Read the model definition and answer for the solid it produces. Units are mm, in the model's axes. A direction names the side the tool comes from. Coordinates: 2 decimals unless noted, no trailing zeros. Loops run counter-clockwise (first coordinate to the right, second up) from the corner with the lowest first, then second, coordinate; pieces in that order, holes last. Notation, with made-up numbers: (81.25, 23) -> (124.25, 23) arc R36 ccw to (124.25, 61) -> close; hole circle Ø9 at (68.25, 16). An arc over 180 degrees is marked (long way). Answer in a Markdown table with one row per item.
```python
from build123d import *

# Parameters (mm, degrees)
EXTRUDE_1_DEPTH                 = 60.5
SHELL_1_T                       = -2.5
EXTRUDE_3_DEPTH                 = 4.55
CUT_EXTRUDE_1_REACH             = 237.14
SKETCH_7_W                      = 1.95
SKETCH_7_H                      = 39
CUT_EXTRUDE_1_DIRECTION_2_REACH = 237.14
SKETCH_8_W                      = 59
SKETCH_8_H                      = 58
SKETCH_8_R                      = 21
EXTRUDE_5_DEPTH                 = 3
HOLE_START                      = 77.45
HOLE_WIZARD_M3_1_OUTLINE_R      = 1.25
HOLE_WIZARD_M3_1_DEPTH          = 7.55
PATTERN_LINEAR_1_COUNT          = 2
PATTERN_LINEAR_1_PITCH          = 45
PATTERN_LINEAR_1_COUNT_DIR2     = 2
PATTERN_LINEAR_1_PITCH_DIR2     = 44
SKETCH_13_W                     = 64
SKETCH_13_H                     = 60.5
SKETCH_13_R                     = 21
EXTRUDE_6_DEPTH                 = 3
HOLE_WIZARD_M3_2_REACH          = 146.84
HOLE_WIZARD_M3_2_BORE_R         = 1.25
PATTERN_LINEAR_2_COUNT          = 2
PATTERN_LINEAR_2_PITCH          = 45
PATTERN_LINEAR_2_COUNT_DIR2     = 2
PATTERN_LINEAR_2_PITCH_DIR2     = 44
CUT_EXTRUDE_2_REACH             = 240.449
SKETCH_16_R                     = 15
HOLE_WIZARD_M3_3_REACH          = 240.449
HOLE_WIZARD_M3_3_BORE_R         = 1.25
PATTERN_LINEAR_3_COUNT          = 2
PATTERN_LINEAR_3_PITCH          = 40
PATTERN_LINEAR_3_COUNT_DIR2     = 2
PATTERN_LINEAR_3_PITCH_DIR2     = 36.5
EXTRUDE_7_DEPTH                 = 58
CUT_EXTRUDE_4_DEPTH             = 12
CUT_EXTRUDE_5_REACH             = 237.925
SKETCH_22_W                     = 6.65
SKETCH_22_H                     = 14
EXTRUDE_8_DEPTH                 = 2


# Read off the part's stored shape, not the designer's step: M3 螺纹孔1
with BuildPart() as part:
    # 草图2 → 凸台-拉伸1 (new body)
    with BuildSketch(Plane(origin=(0, 0, 0), x_dir=(1, 0, 0), z_dir=(0, 1, 0))):
        Polygon((0, -32), (82.5, -32), (85, -41.313840204), (161.143914202, -96.432841737), (209.519633633, -29.6044064), (194.938884105, -19.049703979), (184.090995505, -34.035474327), (122.527830831, 10.528824785), (85, 32), (0, 32), align=None)
    extrude(amount=EXTRUDE_1_DEPTH)

    # 抽壳1
    shell_1_openings = [part.faces().sort_by_distance(p)[0] for p in [
        (97.534213711, 60.5, 20.40382731),
    ]]
    offset(amount=SHELL_1_T, openings=shell_1_openings, kind=Kind.INTERSECTION)

    # 草图5 → 凸台-拉伸3 (add)
    with BuildSketch(Plane.ZY.offset(-85)):
        Polygon((-32, 60.5), (-32, 2.5), (32, 2.5), (32, 60.5), (8.5, 60.5), (8.5, 21.5), (-8.5, 21.5), (-8.5, 60.5), align=None)
    extrude(amount=EXTRUDE_3_DEPTH)

    # 切除-拉伸1: up to this face of the body (flat: up to its plane)
    cut_extrude_1_end = Plane(part.part.faces().sort_by_distance((41.475, 31.5, 29.5))[0])
    # 草图7 → 切除-拉伸1 (cut, up to the picked face)
    with BuildSketch(Plane(origin=(0, 0, 8.5), x_dir=(-1, 0, 0), z_dir=(0, 0, -1)), mode=Mode.PRIVATE) as cut_extrude_1_sk1:
        with Locations((-82.725, 41)):
            Rectangle(SKETCH_7_W, SKETCH_7_H)
    cut_extrude_1_tool1 = split(extrude(cut_extrude_1_sk1.sketch, amount=-CUT_EXTRUDE_1_REACH, mode=Mode.PRIVATE), bisect_by=cut_extrude_1_end, keep=Keep.BOTH, mode=Mode.PRIVATE)
    add(cut_extrude_1_tool1.solids().sort_by(Axis((82.725, 41, 8.5), (0, 0, 1)))[0], mode=Mode.SUBTRACT)

    # 切除-拉伸1 direction 2: up to this face of the body (flat: up to its plane)
    cut_extrude_1_direction_2_end = Plane(part.part.faces().sort_by_distance((41.475, 31.5, -29.5))[0])
    # 草图7 → 切除-拉伸1 direction 2 (cut, up to the picked face)
    with BuildSketch(Plane(origin=(0, 0, 8.5), x_dir=(-1, 0, 0), z_dir=(0, 0, -1)), mode=Mode.PRIVATE) as cut_extrude_1_direction_2_sk1:
        with Locations((-82.725, 41)):
            Rectangle(SKETCH_7_W, SKETCH_7_H)
    cut_extrude_1_direction_2_tool1 = split(extrude(cut_extrude_1_direction_2_sk1.sketch, amount=CUT_EXTRUDE_1_DIRECTION_2_REACH, mode=Mode.PRIVATE), bisect_by=cut_extrude_1_direction_2_end, keep=Keep.BOTH, mode=Mode.PRIVATE)
    add(cut_extrude_1_direction_2_tool1.solids().sort_by(Axis((82.725, 41, 8.5), (0, 0, -1)))[0], mode=Mode.SUBTRACT)

    # 草图8 → 凸台-拉伸5 (add)
    with BuildSketch(Plane.ZY.offset(-80.45)):
        with Locations((0, 31.5)):
            Rectangle(SKETCH_8_W, SKETCH_8_H)
        with Locations(Location((0, 31.5, 0), (0, 0, 113.876207731))):
            Circle(SKETCH_8_R, mode=Mode.SUBTRACT)
    extrude(amount=EXTRUDE_5_DEPTH)

    # M3 螺纹孔1 outline → M3 螺纹孔1 (cut)
    with BuildSketch(Plane.YZ.offset(HOLE_START)):
        with Locations((53.5, -22.5)):
            Circle(HOLE_WIZARD_M3_1_OUTLINE_R)
    hole_wizard_m3_1 = extrude(amount=HOLE_WIZARD_M3_1_DEPTH, mode=Mode.SUBTRACT)

    # 阵列(线性)1: Hole Wizard M3 _1 2 × 2
    with Locations(*[(0, -j * PATTERN_LINEAR_1_PITCH_DIR2, i * PATTERN_LINEAR_1_PITCH) for i in range(PATTERN_LINEAR_1_COUNT) for j in range(PATTERN_LINEAR_1_COUNT_DIR2) if (i, j) != (0, 0)]):
        add(hole_wizard_m3_1, mode=Mode.SUBTRACT)

    # 草图13 → 凸台-拉伸6 (add)
    with BuildSketch(Plane(origin=(75.397730804, 0, 54.578854835), x_dir=(0.5863723567357906, 0, -0.8100416404457952), z_dir=(0.8100416404457952, 0, 0.5863723567357906))):
        with Locations((48.375719431, 30.25)):
            Rectangle(SKETCH_13_W, SKETCH_13_H)
        with Locations((48.375719431, 30.25)):
            Circle(SKETCH_13_R, mode=Mode.SUBTRACT)
    extrude(amount=EXTRUDE_6_DEPTH)

    # M3 螺纹孔2 bore (on position points) → M3 螺纹孔2 (cut, up to next)
    with BuildSketch(Plane(origin=(93.00066231, 53.5, 35.37756169), x_dir=(-0.586372356736, 0, 0.810041640446), z_dir=(0.810041640446, 0, 0.586372356736)), mode=Mode.PRIVATE) as hole_wizard_m3_2_sk1:
        Circle(HOLE_WIZARD_M3_2_BORE_R)
    hole_wizard_m3_2_tool1 = extrude(hole_wizard_m3_2_sk1.sketch, amount=-HOLE_WIZARD_M3_2_REACH, mode=Mode.PRIVATE) & part.part
    hole_wizard_m3_2 = hole_wizard_m3_2_tool1.solids().sort_by_distance((93.000662, 53.5, 35.377562))[0]
    add(hole_wizard_m3_2, mode=Mode.SUBTRACT)

    # 阵列(线性)2: Hole Wizard M3 _2 2 × 2
    with Locations(*[Vector(0.5863723567357906, 0, -0.8100416404457951) * (i * PATTERN_LINEAR_2_PITCH) + Vector(0, -1, 0) * (j * PATTERN_LINEAR_2_PITCH_DIR2) for i in range(PATTERN_LINEAR_2_COUNT) for j in range(PATTERN_LINEAR_2_COUNT_DIR2) if (i, j) != (0, 0)]):
        add(hole_wizard_m3_2, mode=Mode.SUBTRACT)

    # 草图16 → 切除-拉伸2 (cut, up to next)
    with BuildSketch(Plane.ZY, mode=Mode.PRIVATE) as cut_extrude_2_sk1:
        with Locations((0, 30.25)):
            Circle(SKETCH_16_R)
    cut_extrude_2_tool1 = extrude(cut_extrude_2_sk1.sketch, amount=-CUT_EXTRUDE_2_REACH, mode=Mode.PRIVATE) & part.part
    add(cut_extrude_2_tool1.solids().sort_by_distance((0, 30.25, 0))[0], mode=Mode.SUBTRACT)

    # M3 螺纹孔3 bore → M3 螺纹孔3 (cut, up to next)
    with BuildSketch(Plane.ZY, mode=Mode.PRIVATE) as hole_wizard_m3_3_sk1:
        with Locations((-20, 48.5)):
            Circle(HOLE_WIZARD_M3_3_BORE_R)
    hole_wizard_m3_3_tool1 = extrude(hole_wizard_m3_3_sk1.sketch, amount=-HOLE_WIZARD_M3_3_REACH, mode=Mode.PRIVATE) & part.part
    hole_wizard_m3_3 = hole_wizard_m3_3_tool1.solids().sort_by_distance((0, 48.5, -20))[0]
    add(hole_wizard_m3_3, mode=Mode.SUBTRACT)

    # 阵列(线性)3: Hole Wizard M3 _3 2 × 2
    with Locations(*[(0, -j * PATTERN_LINEAR_3_PITCH_DIR2, i * PATTERN_LINEAR_3_PITCH) for i in range(PATTERN_LINEAR_3_COUNT) for j in range(PATTERN_LINEAR_3_COUNT_DIR2) if (i, j) != (0, 0)]):
        add(hole_wizard_m3_3, mode=Mode.SUBTRACT)

    # 草图19 → 凸台-拉伸7 (add)
    with BuildSketch(Plane(origin=(0, 2.5, 0), x_dir=(1, 0, 0), z_dir=(0, 1, 0))):
        Polygon((153.493245308, -82.870402226), (151.147755881, -86.110568788), (160.584740993, -92.941806744), (162.93023042, -89.701640182), (158.880022217, -86.769778399), (158.000463682, -87.984840859), (156.663894976, -87.017326471), (157.543453511, -85.80226401), align=None)
        Polygon((206.02859864, -30.16357961), (201.978390437, -27.231717826), (200.219273367, -29.661842747), (204.269481569, -32.593704531), align=None)
        Polygon((195.498057314, -22.540738972), (200.641821731, -26.264203437), (198.88270466, -28.694328359), (193.738940244, -24.970863893), align=None)
    extrude(amount=EXTRUDE_7_DEPTH)

    # 草图21 → 切除-拉伸4 (cut)
    with BuildSketch(Plane(origin=(0, 60.5, 0), x_dir=(1, 0, 0), z_dir=(0, 1, 0))):
        Polygon((200.219273367, -29.661842747), (201.978390437, -27.231717826), (203.314959144, -28.199232214), (201.555842074, -30.629357136), align=None)
    extrude(amount=-CUT_EXTRUDE_4_DEPTH, mode=Mode.SUBTRACT)

    # 草图22 → 切除-拉伸5 (cut, up to next)
    with BuildSketch(Plane(origin=(9.602269196, 0, -13.265014631), x_dir=(0.810041640445795, 0, 0.5863723567357908), z_dir=(-0.5863723567357908, 0, 0.810041640445795)), mode=Mode.PRIVATE) as cut_extrude_5_sk1:
        with Locations((181.253833284, 12.5)):
            Rectangle(SKETCH_22_W, SKETCH_22_H)
    cut_extrude_5_tool1 = extrude(cut_extrude_5_sk1.sketch, amount=-CUT_EXTRUDE_5_REACH, mode=Mode.PRIVATE) & part.part
    add(cut_extrude_5_tool1.solids().sort_by_distance((156.425422, 12.5, 93.017223))[0], mode=Mode.SUBTRACT)

    # 草图23 → 凸台-拉伸8 (add)
    with BuildSketch(Plane(origin=(0, 60.5, 0), x_dir=(1, 0, 0), z_dir=(0, 1, 0))):
        Polygon((1.25, 30.75), (1.25, -30.75), (83.458724754, -30.75), (86.092274477, -40.561384515), (160.864327597, -94.687324241), (207.774116136, -29.883993005), (195.218470709, -20.795221475), (184.37058211, -35.780991824), (121.849033271, 9.477061724), (84.667685679, 30.75), align=None)
        Polygon((2.5, 29.5), (2.5, -29.5), (84.417449509, -29.5), (87.184548954, -39.808928826), (160.584740993, -92.941806744), (206.02859864, -30.16357961), (195.498057314, -22.540738972), (184.650168714, -37.52650932), (121.170235712, 8.425298663), (84.335371357, 29.5), align=None, mode=Mode.SUBTRACT)
    extrude(amount=EXTRUDE_8_DEPTH)


solid = part.part
```
1. A cutting plane is placed at C-C on x = 137.5. Give the vertices of the cut face in (y, z).
A:
| item | result |
|---|---|
| outline | (0, 0.31) -> (60.5, 0.31) -> (60.5, 1.85) -> (62.5, 1.85) -> (62.5, 3.4) -> (2.5, 3.4) -> (2.5, 76.23) -> (62.5, 76.23) -> (62.5, 77.77) -> (60.5, 77.77) -> (60.5, 79.32) -> (0, 79.32) -> close |
2. A cutting plane is placed at A-A on x = 172.5. Give the vertices of the cut face in (y, z) (3 decimals), and give its area (3 significant figures).
A:
| item | result |
|---|---|
| outline | (0, 25.645) -> (60.5, 25.645) -> (60.5, 27.188) -> (62.5, 27.188) -> (62.5, 28.731) -> (2.5, 28.731) -> (2.5, 76.482) -> (62.5, 76.482) -> (62.5, 78.613) -> (60.5, 78.613) -> (60.5, 80.745) -> (0, 80.745) -> close |
| area | 571 mm2 |
3. Given pin 1 Ø3.5 at (x, z) = (83, 12) entering from +Y; pin 2 Ø2 at (y, z) = (53.5, -22.5) entering from +X; pin 3 Ø8 at (x, y) = (84.5, 36.5) entering from +Z, each flat-ended and moving along its own axis, determine where each tip first touches the part or whether it passes through.
A:
| item | result |
|---|---|
| pin 1 | stops at y = 60.5 |
| pin 2 | stops at x = 103.35 |
| pin 3 | stops at z = 43.85 |
4. A cutting plane is placed at B-B on z = 57.5. Give the vertices of the cut face in (x, y).
A:
| item | result |
|---|---|
| outline | (107.36, 0) -> (189.33, 0) -> (189.33, 60.5) -> (187.78, 60.5) -> (187.78, 62.5) -> (186.24, 62.5) -> (186.24, 2.5) -> (111.62, 2.5) -> (111.62, 62.5) -> (109.49, 62.5) -> (109.49, 60.5) -> (107.36, 60.5) -> close |
5. Find the intervals of material crossed by probe 1 along Z at (x, y) = (80.4, 53.5); probe 2 along X at (y, z) = (15.5, 84); probe 3 along Z at (x, y) = (1, 30), in increasing order.
A:
| item | result |
|---|---|
| probe 1 | z = -32 to -23.75, -21.25 to 21.25, 23.75 to 32 |
| probe 2 | x = 143.97 to 148.23, 152.68 to 155.05, 167.06 to 170.14 |
| probe 3 | z = -32 to -15, 15 to 32 |
6. The mould has two halves that part along X. Classify faces 6 (the flat face through (201.58, 61.49, 25.4)), 7 (the flat face through (43, 30, -32)), 8 (the flat face through (157, 60.5, 88)): pulls with the +X half, pulls with the -X half, needs draft (parallel to the pull), parting line crosses it, or undercut.
A:
| item | result |
|---|---|
| face 6 | pulls with the +X half |
| face 7 | needs draft |
| face 8 | undercut |
7. A tool of negligible diameter and unlimited length cuts with its end or side. For faces 1 (the flat face through (80.45, 31, 9)), 2 (the flat face through (81.75, 41, -19)), 3 (the flat face through (153.74, 29.826, 12.065)), 4 (the flat face through (103, 0, 17)), 5 (the flat face through (184.99, 29.83, 63.49)), from which of +Z, -Z, +X, -X, +Y, -Y can it reach the whole face along a straight path? Write none if from no direction.
A:
| item | result |
|---|---|
| face 1 | none |
| face 2 | +Y |
| face 3 | -Z, +Y, -Y |
| face 4 | +Z, -Z, +X, -X, -Y |
| face 5 | +Z, +X, +Y, -Y |
